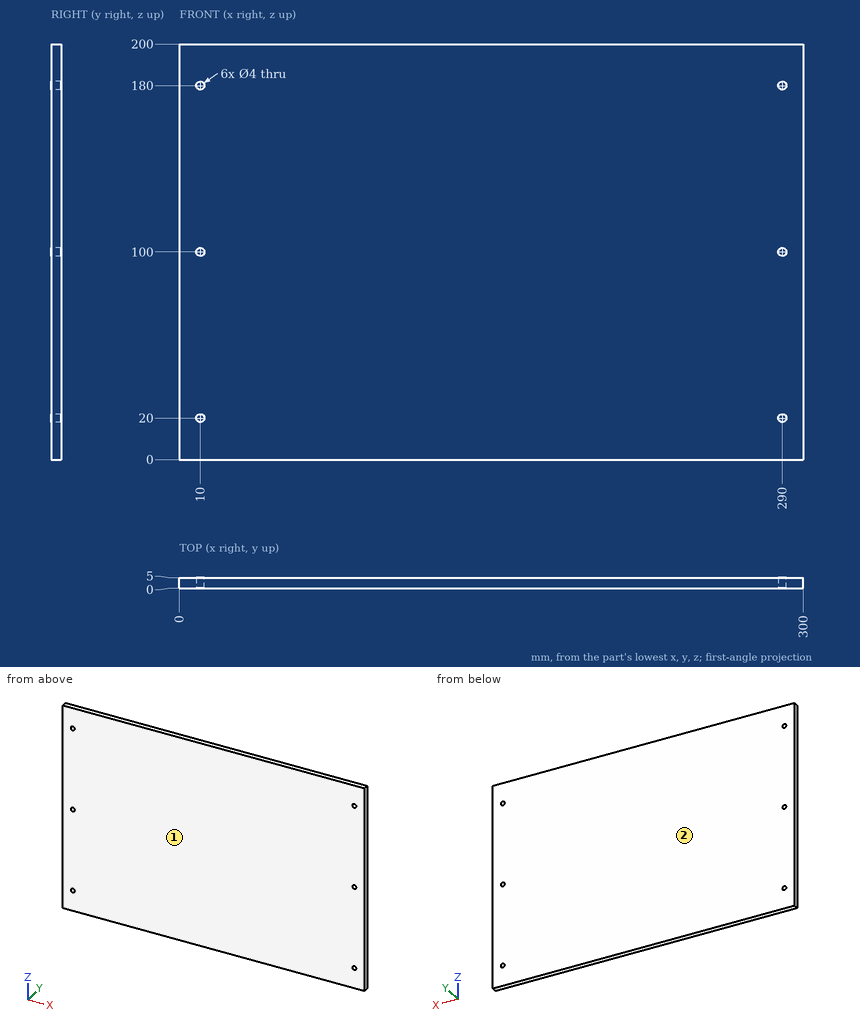
Source: three-view drawing plus pictorial views. Frame: mm from the lowest corner of the part. Coordinates: 2 decimals unless noted, no trailing zeros. Write each question's results on one line, items separated by ' | '. Start each with the question number.
Q1. Pull-direction query (Y, two-part tool) for the marked faces 1 and 2; classes: released by +Y, released by -Y, zero draft, split by the parting line, or undercut.
Q2. Ray query, line 1 (Z direction, x = 10, y = 1); line 2 (X direction, y = 2.5, z = 20). Return the intervals inside material, ascending. Write a range as from..to.
Q3. Pin query (flat end, axial travel): pin 1 (1 mm diameter, centred on x = 243, z = 35, fed in from -Y). Return the tip coordinate at first contact, or that it passes through.
Found:
1) face 1: released by -Y | face 2: released by +Y
2) line 1: 0..18, 22..98, 102..178, 182..200 | line 2: 0..8, 12..288, 292..300
3) pin 1: y = 0
